Build history of the part. All positions in model axes, mm. Face numbers are marked on the shaded views. A direction names the side the tool comes from. Round coordinates to 2 decimals unless told otherwise and drop trailing zeros. Write each loop counter-clockwise with the first axis right and the second up, starting at its lowest first coordinate (ties: lowest second). Pieces come first, ordered by that corner, then holes. Notation, with made-up numbers: (37.5, -0.5) -> (96.5, -0.5) arc R16 cw to (96.5, 18.5) -> close; hole circle Ø4 at (22, -24.5). An arc over 180 degrees is marked (long way). Answer as CSV lines item,"result".
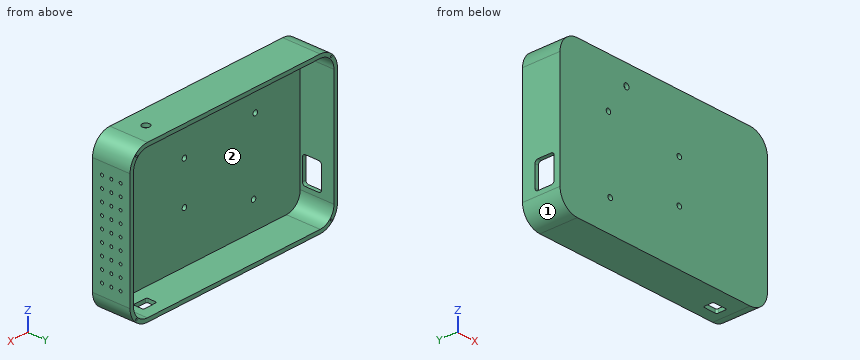
from build123d import *

# Parameters (mm, degrees)
BOSS_EXTRUDE1_DEPTH = 25.4
CUT_EXTRUDE6_DEPTH  = 22.86
SKETCH7_R           = 0.6
CUT_EXTRUDE8_DEPTH  = 2.46
CUT_EXTRUDE9_DEPTH  = 10
SKETCH12_R          = 1
CUT_EXTRUDE10_DEPTH = 10
CUT_EXTRUDE12_DEPTH = 10
SKETCH14_R          = 1.663741232
CUT_EXTRUDE13_DEPTH = 95.390993214
SKETCH15_R          = 1.925
CUT_EXTRUDE14_DEPTH = 95.390993214
SKETCH16_R          = 2.54
CUT_EXTRUDE15_DEPTH = 5.08


with BuildPart() as part:
    # Sketch1 → Boss-Extrude1 (new body)
    with BuildSketch(Plane(origin=(0, 0, 0), x_dir=(1, 0, 0), z_dir=(0, 1, 0))):
        with BuildLine():
            Line((63.5, 50.8), (-63.5, 50.8))
            ThreePointArc((-63.5, 50.8), (-72.480256121, 47.080256121), (-76.2, 38.1))
            Line((-76.2, 38.1), (-76.2, -38.1))
            ThreePointArc((-76.2, -38.1), (-72.480256121, -47.080256121), (-63.5, -50.8))
            Line((-63.5, -50.8), (63.5, -50.8))
            ThreePointArc((63.5, -50.8), (72.480256121, -47.080256121), (76.2, -38.1))
            Line((76.2, -38.1), (76.2, 38.1))
            ThreePointArc((76.2, 38.1), (72.480256121, 47.080256121), (63.5, 50.8))
        make_face()
    extrude(amount=BOSS_EXTRUDE1_DEPTH)

    # Sketch4 → Cut-Extrude6 (cut)
    with BuildSketch(Plane(origin=(0, 25.4, 0), x_dir=(1, 0, 0), z_dir=(0, 1, 0))):
        with BuildLine():
            Line((-63.5, 48.26), (63.5, 48.26))
            ThreePointArc((63.5, 48.26), (70.684204897, 45.284204897), (73.66, 38.1))
            Line((73.66, 38.1), (73.66, -38.1))
            ThreePointArc((73.66, -38.1), (70.684204897, -45.284204897), (63.5, -48.26))
            Line((63.5, -48.26), (-63.5, -48.26))
            ThreePointArc((-63.5, -48.26), (-70.684204897, -45.284204897), (-73.66, -38.1))
            Line((-73.66, -38.1), (-73.66, 38.1))
            ThreePointArc((-73.66, 38.1), (-70.684204897, 45.284204897), (-63.5, 48.26))
        make_face()
    extrude(amount=-CUT_EXTRUDE6_DEPTH, mode=Mode.SUBTRACT)

    # Sketch7 → Cut-Extrude8 (cut)
    with BuildSketch(Plane(origin=(0, 25.4, 0), x_dir=(1, 0, 0), z_dir=(0, 1, 0))):
        with Locations(Location((-71.56, 46.16, 0), (0, 0, 270))):
            Circle(SKETCH7_R)
        with Locations(Location((-71.56, -46.16, 0), (0, 0, 270))):
            Circle(SKETCH7_R)
        with Locations(Location((71.56, -46.16, 0), (0, 0, 270))):
            Circle(SKETCH7_R)
        with Locations(Location((71.56, 46.16, 0), (0, 0, 270))):
            Circle(SKETCH7_R)
    extrude(amount=-CUT_EXTRUDE8_DEPTH, mode=Mode.SUBTRACT)

    # Sketch10 → Cut-Extrude9 (cut)
    with BuildSketch(Plane.ZY.offset(76.2)):
        with BuildLine():
            Line((-33.1, 17), (-19.1, 17))
            ThreePointArc((-19.1, 17), (-17.685786438, 16.414213562), (-17.1, 15))
            Line((-17.1, 15), (-17.1, 6))
            ThreePointArc((-17.1, 6), (-17.685786438, 4.585786438), (-19.1, 4))
            Line((-19.1, 4), (-33.1, 4))
            ThreePointArc((-33.1, 4), (-34.514213562, 4.585786438), (-35.1, 6))
            Line((-35.1, 6), (-35.1, 15))
            ThreePointArc((-35.1, 15), (-34.514213562, 16.414213562), (-33.1, 17))
        make_face()
    extrude(amount=-CUT_EXTRUDE9_DEPTH, mode=Mode.SUBTRACT)

    # Sketch12 → Cut-Extrude10 (cut)
    with BuildSketch(Plane(origin=(76.2, 0, 0), x_dir=(0, 0, -1), z_dir=(1, 0, 0))):
        with Locations((-30.48, 19)):
            Circle(SKETCH12_R)
        with Locations((-30.48, 12.7)):
            Circle(SKETCH12_R)
        with Locations((-30.48, 6.4)):
            Circle(SKETCH12_R)
        with Locations((-22.86, 19)):
            Circle(SKETCH12_R)
        with Locations((-22.86, 12.7)):
            Circle(SKETCH12_R)
        with Locations((-22.86, 6.4)):
            Circle(SKETCH12_R)
        with Locations((-15.24, 19)):
            Circle(SKETCH12_R)
        with Locations((-15.24, 12.7)):
            Circle(SKETCH12_R)
        with Locations((-15.24, 6.4)):
            Circle(SKETCH12_R)
        with Locations((-7.62, 19)):
            Circle(SKETCH12_R)
        with Locations((-7.62, 12.7)):
            Circle(SKETCH12_R)
        with Locations((-7.62, 6.4)):
            Circle(SKETCH12_R)
        with Locations((0, 19)):
            Circle(SKETCH12_R)
        with Locations((0, 12.7)):
            Circle(SKETCH12_R)
        with Locations((0, 6.4)):
            Circle(SKETCH12_R)
        with Locations((7.62, 19)):
            Circle(SKETCH12_R)
        with Locations((7.62, 12.7)):
            Circle(SKETCH12_R)
        with Locations((7.62, 6.4)):
            Circle(SKETCH12_R)
        with Locations((15.24, 19)):
            Circle(SKETCH12_R)
        with Locations((15.24, 12.7)):
            Circle(SKETCH12_R)
        with Locations((15.24, 6.4)):
            Circle(SKETCH12_R)
        with Locations((22.86, 19)):
            Circle(SKETCH12_R)
        with Locations((22.86, 12.7)):
            Circle(SKETCH12_R)
        with Locations((22.86, 6.4)):
            Circle(SKETCH12_R)
        with Locations((30.48, 19)):
            Circle(SKETCH12_R)
        with Locations((30.48, 12.7)):
            Circle(SKETCH12_R)
        with Locations((30.48, 6.4)):
            Circle(SKETCH12_R)
    extrude(amount=-CUT_EXTRUDE10_DEPTH, mode=Mode.SUBTRACT)

    # Sketch13 → Cut-Extrude12 (cut)
    with BuildSketch(Plane(origin=(0, 0, -50.8), x_dir=(-1, 0, 0), z_dir=(0, 0, -1))):
        with BuildLine():
            Line((-57.2, 17.839671087), (-49.2, 17.839671087))
            ThreePointArc((-49.2, 17.839671087), (-48.492893219, 17.546777868), (-48.2, 16.839671087))
            Line((-48.2, 16.839671087), (-48.2, 11.839671087))
            ThreePointArc((-48.2, 11.839671087), (-48.492893219, 11.132564306), (-49.2, 10.839671087))
            Line((-49.2, 10.839671087), (-57.2, 10.839671087))
            ThreePointArc((-57.2, 10.839671087), (-57.907106781, 11.132564306), (-58.2, 11.839671087))
            Line((-58.2, 11.839671087), (-58.2, 16.839671087))
            ThreePointArc((-58.2, 16.839671087), (-57.907106781, 17.546777868), (-57.2, 17.839671087))
        make_face()
    extrude(amount=-CUT_EXTRUDE12_DEPTH, mode=Mode.SUBTRACT)

    # Sketch14 → Cut-Extrude13 (cut, through all)
    with BuildSketch(Plane(origin=(0, 2.54, 0), x_dir=(1, 0, 0), z_dir=(0, 1, 0))):
        with Locations(Location((-39.37, 30, 0), (0, 0, 270))):
            Circle(SKETCH14_R)
        with Locations(Location((-40.64, -18.26, 0), (0, 0, 270))):
            Circle(SKETCH14_R)
        with Locations(Location((11.43, -13.18, 0), (0, 0, 270))):
            Circle(SKETCH14_R)
        with Locations(Location((11.43, 14.76, 0), (0, 0, 270))):
            Circle(SKETCH14_R)
    extrude(amount=-CUT_EXTRUDE13_DEPTH, mode=Mode.SUBTRACT)

    # Sketch15 → Cut-Extrude14 (cut, through all)
    with BuildSketch(Plane(origin=(0, 2.54, 0), x_dir=(1, 0, 0), z_dir=(0, 1, 0))):
        with Locations(Location((-27.451730326, -37.489635759, 0), (0, 0, 270))):
            Circle(SKETCH15_R)
    extrude(amount=-CUT_EXTRUDE14_DEPTH, mode=Mode.SUBTRACT)

    # Sketch16 → Cut-Extrude15 (cut)
    with BuildSketch(Plane.XY.offset(50.8)):
        with Locations((50.8, 12.7)):
            Circle(SKETCH16_R)
    extrude(amount=-CUT_EXTRUDE15_DEPTH, mode=Mode.SUBTRACT)


solid = part.part
1. Which spindle directions (+Z, -Z, +X, -X, +Y, -Y) get a long thin tool onto all of the face, cutting with end or side? Do the marked faces 1 and 2. Say none if no direction does.
Results found:
face 1,"-Z, -X, +Y, -Y"
face 2,"+Y"
2. Drop flat-ended pins along their axis: pin 1 Ø4.5 at (x, z) = (11.43, 13.18) entering from +Y; pin 2 Ø1.2 at (y, z) = (19, -22.86) entering from +X; pin 3 Ø1.2 at (y, z) = (6.4, -30.48) entering from -X; pin 4 Ø1.3 at (x, y) = (-75, 9) entering from +Z. Give the stop position or say it passes through.
Results found:
pin 1,"stops at y = 2.54"
pin 2,"stops at x = -73.66"
pin 3,"passes through"
pin 4,"stops at z = 44.7"
3. Cut at A-A, the plane z = 18.26. Write the cut outline in (x, y), then the cut area to 3 significant figures.
Results found:
outline,"(-76.2, 0) -> (-42.3, 0) -> (-42.3, 2.54) -> (-73.66, 2.54) -> (-73.66, 25.4) -> (-76.2, 25.4) -> close; (-38.98, 0) -> (76.2, 0) -> (76.2, 25.4) -> (73.66, 25.4) -> (73.66, 2.54) -> (-38.98, 2.54) -> close"
area,"495 mm2"
4. Cut at B-B, the plane x = 11.43. Write the cut outline in (y, z).
Results found:
outline,"(0, -50.8) -> (25.4, -50.8) -> (25.4, -48.26) -> (2.54, -48.26) -> (2.54, -16.42) -> (0, -16.42) -> close; (0, -13.1) -> (2.54, -13.1) -> (2.54, 11.52) -> (0, 11.52) -> close; (0, 14.84) -> (2.54, 14.84) -> (2.54, 48.26) -> (25.4, 48.26) -> (25.4, 50.8) -> (0, 50.8) -> close"
5. Cut at C-C, the plane z = -5. Write the cut outline in (x, y).
Results found:
outline,"(-76.2, 0) -> (76.2, 0) -> (76.2, 25.4) -> (73.66, 25.4) -> (73.66, 2.54) -> (-73.66, 2.54) -> (-73.66, 25.4) -> (-76.2, 25.4) -> close"
6. Probe line 1 along Y through (x, z) = (74.65, 22.86); line 2 along X through (y, z) = (20.5, -35); line 3 along Z through (x, y) = (48, 3.75). List the from-to ranges inside material, lowest first.
Results found:
line 1,"y = 0 to 5.4, 7.4 to 11.7, 13.7 to 18, 20 to 25.4"
line 2,"x = -76.2 to -73.66, 73.66 to 76.2"
line 3,"z = -50.8 to -48.26, 48.26 to 50.8"
